```python
from build123d import *

# Parameters (mm, degrees)
BOSS_EXTRUDE1_DEPTH     = 5
SKETCH2_R               = 4
BOSS_EXTRUDE2_DEPTH     = 10
SKETCH6_R               = 4
BOSS_EXTRUDE3_DEPTH     = 10
MIRROR2_COPY_1_SKETCH_R = 4
MIRROR2_COPY_1_DEPTH    = 10
MIRROR2_COPY_3_SKETCH_R = 4
MIRROR2_COPY_3_DEPTH    = 10


with BuildPart() as part:
    # Sketch1 → Boss-Extrude1 (new, symmetric)
    with BuildSketch(Plane(origin=(0, 0, 0), x_dir=(1, 0, 0), z_dir=(0, 1, 0))):
        Polygon((5, 8.660254038), (-5, 8.660254038), (-10, 0), (-5, -8.660254038), (5, -8.660254038), (10, 0), align=None)
        Polygon((-7.113248654, 0), (-3.556624327, -6.160254038), (3.556624327, -6.160254038), (7.113248654, 0), (3.556624327, 6.160254038), (-3.556624327, 6.160254038), align=None, mode=Mode.SUBTRACT)
    extrude(amount=BOSS_EXTRUDE1_DEPTH, both=True)

    # Sketch2 → Boss-Extrude2 (add)
    with BuildSketch(Plane(origin=(0, 0, -8.660254038), x_dir=(-1, 0, 0), z_dir=(0, 0, -1))):
        Circle(SKETCH2_R)
    extrude(amount=BOSS_EXTRUDE2_DEPTH)

    # Sketch3 → Revolve1 (revolve)
    with BuildSketch(Plane(origin=(0, 0, 0), x_dir=(0, 0, -1), z_dir=(1, 0, 0)), mode=Mode.PRIVATE) as revolve1_sk:
        Polygon((18.660254038, 4), (22.560254038, 0.1), (22.560254038, 0), (18.660254038, 0), align=None)
    revolve(revolve1_sk.sketch.rotate(Axis((0, 0, 981.339745962), (0, 0, -1)), 90), axis=Axis((0, 0, 981.339745962), (0, 0, -1)))

    # Sketch6 → Boss-Extrude3 (add)
    with BuildSketch(Plane(origin=(7.5, 0, -4.330127019), x_dir=(-0.49999999999999983, 0, -0.8660254037844388), z_dir=(0.8660254037844387, 0, -0.4999999999999998))):
        with Locations(Location((0, 0, 0), (0, 0, 180))):
            Circle(SKETCH6_R)
    boss_extrude3 = extrude(amount=BOSS_EXTRUDE3_DEPTH)

    # Sketch9 → Revolve4 (revolve)
    with BuildSketch(Plane(origin=(0, 0, 0), x_dir=(1, 0, 0), z_dir=(0, 1, 0)), mode=Mode.PRIVATE) as revolve4_sk:
        Polygon((14.160254038, 12.794228634), (19.487753113, 11.366729559), (19.537753113, 11.280127019), (16.160254038, 9.330127019), align=None)
    revolve4 = revolve(revolve4_sk.sketch.rotate(Axis((0, 0, 0), (0.8660254037844387, 0, -0.5000000000000001)), 180), axis=Axis((0, 0, 0), (0.8660254037844387, 0, -0.5000000000000001)))

    # Sketch10 → Revolve5 (revolve)
    with BuildSketch(Plane(origin=(0, 0, 0), x_dir=(1, 0, 0), z_dir=(0, 1, 0)), mode=Mode.PRIVATE) as revolve5_sk:
        Polygon((9.5, -0.866025404), (18.160254038, -5.866025404), (19.587753113, -11.193524479), (19.537753113, -11.280127019), (7.5, -4.330127019), align=None)
    revolve5 = revolve(revolve5_sk.sketch.rotate(Axis((0, 0, 0), (0.8660254037844387, 0, 0.5)), 180), axis=Axis((0, 0, 0), (0.8660254037844387, 0, 0.5)))

    # Mirror1: Boss-Extrude3, Revolve4 across plane
    add(boss_extrude3.mirror(Plane(origin=(0, 0, 0), x_dir=(0.49999999999999983, 0, 0.8660254037844387), z_dir=(0.8660254037844388, 0, -0.49999999999999983))))
    add(revolve4.mirror(Plane(origin=(0, 0, 0), x_dir=(0.49999999999999983, 0, 0.8660254037844387), z_dir=(0.8660254037844388, 0, -0.49999999999999983))))

    # Mirror2: Revolve5 across plane
    add(revolve5.mirror(Plane(origin=(0, 0, 0), x_dir=(-0.49999999999999983, 0, 0.8660254037844387), z_dir=(0.8660254037844388, 0, 0.49999999999999983))))

    # Mirror2 copy 1 sketch → Mirror2 copy 1 (add)
    with BuildSketch(Plane.XY.offset(8.660254038)):
        with Locations(Location((0, 0, 0), (0, 0, 180))):
            Circle(MIRROR2_COPY_1_SKETCH_R)
    extrude(amount=MIRROR2_COPY_1_DEPTH)

    # Mirror2 copy 2 sketch → Mirror2 copy 2 (revolve)
    with BuildSketch(Plane(origin=(0, 0, 0), x_dir=(-0.499999999999999, 0, 0.8660254037844393), z_dir=(0, 1, 0))):
        Polygon((14.160254038, 12.794228634), (19.487753113, 11.366729559), (19.537753113, 11.280127019), (16.160254038, 9.330127019), align=None)
    revolve(axis=Axis((0, 0, 0), (0, 0, 1)))

    # Mirror2 copy 3 sketch → Mirror2 copy 3 (add)
    with BuildSketch(Plane(origin=(0, 0, -8.660254038), x_dir=(1, 0, 0), z_dir=(0, 0, -1))):
        Circle(MIRROR2_COPY_3_SKETCH_R)
    extrude(amount=MIRROR2_COPY_3_DEPTH)

    # Mirror2 copy 4 sketch → Mirror2 copy 4 (revolve)
    with BuildSketch(Plane(origin=(0, 0, 0), x_dir=(-0.5000000000000007, 0, -0.8660254037844385), z_dir=(0, 1, 0))):
        Polygon((14.160254038, -12.794228634), (19.487753113, -11.366729559), (19.537753113, -11.280127019), (16.160254038, -9.330127019), align=None)
    revolve(axis=Axis((0, 0, 0), (0, 0, 1)))


solid = part.part
```
Here's how the part is built. I have some questions about the finished solid (model axes, mm). A direction names the side the tool comes from. Round coordinates to 2 decimals unless told otherwise and drop trailing zeros. Order: outer loops, then holes, each group sorted by start corner. A loop starts at its lowest first (then second) coordinate and runs counter-clockwise, first axis right, second up. Notation, with made-up numbers: (81.5, 13) -> (95.5, 13) arc R33 cw to (95.5, 49) -> close; hole circle Ø7 at (41, 78). An arc over 180 degrees is marked (long way). Use a Markdown table: item, result. Add a question column.
(1) If we mould it in two halves opening along X, with no side actions, what happens to faces 4 (the face through (0.867, 3.905, 13.59)), 5 (the face through (0.867, -3.905, -13.59)), 6 (the face through (-19.16, 0.44, -9.83)), 7 (the face through (1.103, 0.347, 21.504))? For each: released by +X, released by -X, zero draft, split by the parting line, or undercut.
(2) Suppose I cut it at B-B, the plane z = -18. Please give me the cut outline in (x, y), and give its area (3 significant figures).
(3) I need wall thicknesses on line 1 along X through (y, z) = (-2.5, 0); line 2 along X through (y, z) = (0.75, -9); line 3 along Y through (x, z) = (-15.5, 9). Which ranges of each line are inside material? Lowest first, please.
(4) For faces 1 (the face through (5.31, 0.07, 3.12)), 2 (the face through (4.5, 0.1, -8.66)), 3 (the face through (7.535, 4.514, -4.27)), which set-ups out of +Z, -Z, +X, -X, +Y, -Y let a thin tool reach every point of the face, with its end or its side?
(5) For pin 1 Ø1.5 at (y, z) = (4, 17) entering from -X; pin 2 Ø3 at (x, y) = (0, -3) entering from +Z; pin 3 Ø5 at (x, y) = (13.5, 2.5) entering from -Z, each with a flat end and sliding along its axis, tell me the tip position at first contact or that it passes through.
(6) Suppose I cut it at A-A, the plane z = 10. Count the separate pieces of the cut face and the enclosed holes in it, and give its area (3 significant figures).
Verdict:
| question | item | result |
|---|---|---|
| 1 | face 4 | undercut |
| 1 | face 5 | undercut |
| 1 | face 6 | released by -X |
| 1 | face 7 | split by the parting line |
| 2 | outline | circle Ø8 at (0, 0) |
| 2 | area | 50.3 mm2 |
| 3 | line 1 | -10 to -7.11, 7.11 to 10 |
| 3 | line 2 | -18.88 to -7.73, -3.93 to 3.93, 7.73 to 18.88 |
| 3 | line 3 | -4 to 4 |
| 4 | face 1 | +Y, -Y |
| 4 | face 2 | -Z |
| 4 | face 3 | none |
| 5 | pin 1 | x = -2.33 |
| 5 | pin 2 | z = 21.16 |
| 5 | pin 3 | z = -12.79 |
| 6 | separate pieces | 3 |
| 6 | enclosed holes | 0 |
| 6 | area | 160 mm2 |
